Could you check a few things on this model? Use its own coordinates, in mm. A direction names the side the tool comes from. Coordinates: 2 decimals unless noted, no trailing zeros. Order: outer loops, then holes, each group sorted by start corner. A loop starts at its lowest first (then second) coordinate and runs counter-clockwise, first axis right, second up. Notation, with made-up numbers: (59.25, 54.25) - (82.25, 54.25) arc R17 cw to (82.25, 60.25) - close; hole circle Ø5 at (-37, -39.5). An arc over 180 degrees is marked (long way). One line per item, written item: value.
from build123d import *

# Parameters (mm, degrees)
SKETCH1_R                     = 43.815
HOUSING_FITTING_EXTRUDE_DEPTH = 17.018
HOUSING_BODY_1_DEPTH          = 25.4
SKETCH3_R                     = 6.3754
IMPELLER_BORE_DEPTH           = 17.018
O_RING_CUT_DEPTH              = 1.27
O_RING_CUT_DEPTH_BACK         = 1.27
SKETCH5_R                     = 43.942
SKETCH5_R_2                   = 43.18
SKETCH14_R                    = 3.3734375
CUT_EXTRUDE4_DEPTH            = 19.05
SKETCH15_R                    = 3.3734375
CUT_EXTRUDE5_DEPTH            = 19.05
FILLET1_R                     = 6.604
SKETCH20_R                    = 60.96
SKETCH20_R_2                  = 43.815
BOSS_EXTRUDE1_DEPTH           = 3.175
SKETCH21_R                    = 60.96
SKETCH21_R_2                  = 57.15
BOSS_EXTRUDE2_DEPTH           = 38.1
SKETCH23_R                    = 50.00625
SKETCH23_R_2                  = 43.815
BOSS_EXTRUDE3_DEPTH           = 13.843
SKETCH25_R                    = 3.3734375
CUT_EXTRUDE13_DEPTH           = 25.4
SKETCH26_R                    = 12.954
CUT_EXTRUDE14_DEPTH           = 25.908
SKETCH29_R                    = 45.72
SKETCH29_R_2                  = 44.45
SKETCH29_R_3                  = 43.18
SKETCH29_R_4                  = 41.91
SKETCH29_R_5                  = 40.64
SKETCH29_R_6                  = 39.37
SKETCH29_R_7                  = 38.1
SKETCH29_R_8                  = 36.83
SKETCH29_R_9                  = 35.56
SKETCH29_R_10                 = 34.29
SKETCH29_R_11                 = 33.02
SKETCH29_R_12                 = 31.75
SKETCH29_R_13                 = 30.48
SKETCH29_R_14                 = 29.21
SKETCH29_R_15                 = 27.94
SKETCH29_R_16                 = 26.67
SKETCH29_R_17                 = 25.4
CUT_EXTRUDE16_DEPTH           = 1.5875


with BuildPart() as part:
    # Sketch1 → Housing Fitting Extrude (new body)
    with BuildSketch(Plane(origin=(0, 0, 0), x_dir=(0, 0, -1), z_dir=(1, 0, 0))):
        Circle(SKETCH1_R)
    extrude(amount=HOUSING_FITTING_EXTRUDE_DEPTH)

    # Sketch2 → Housing Body 1 (add)
    with BuildSketch(Plane.ZY):
        with BuildLine():
            Line((60.96, 0), (60.96, 60.96))
            Line((60.96, 60.96), (0, 60.96))
            ThreePointArc((0, 60.96), (-43.105229381, 43.105229381), (-60.96, 0))
            Line((-60.96, 0), (-60.96, -54.61))
            Line((-60.96, -54.61), (-60.96, -60.96))
            Line((-60.96, -60.96), (60.96, -60.96))
            Line((60.96, -60.96), (60.96, -54.61))
            Line((60.96, -54.61), (60.96, 0))
        make_face()
    extrude(amount=HOUSING_BODY_1_DEPTH)

    # Sketch3 → Impeller Bore (cut)
    with BuildSketch(Plane(origin=(17.018, 0, 0), x_dir=(0, 0, -1), z_dir=(1, 0, 0))):
        Circle(SKETCH3_R)
    extrude(amount=-IMPELLER_BORE_DEPTH, mode=Mode.SUBTRACT)

    # Sketch5 → O-Ring Cut (cut, two sides: drawn at the far end of the back side and taken through both)
    with BuildSketch(Plane(origin=(8.509, 0, 0), x_dir=(0, 0, -1), z_dir=(1, 0, 0)).offset(-O_RING_CUT_DEPTH_BACK)):
        Circle(SKETCH5_R)
        Circle(SKETCH5_R_2, mode=Mode.SUBTRACT)
    extrude(amount=O_RING_CUT_DEPTH + O_RING_CUT_DEPTH_BACK, mode=Mode.SUBTRACT)

    # Sketch14 → Cut-Extrude4 (cut)
    with BuildSketch(Plane.XZ.offset(60.96)):
        with Locations(Location((-9.525, -41.91, 0), (0, 0, 270))):
            Circle(SKETCH14_R)
        with Locations(Location((-9.525, 41.91, 0), (0, 0, 270))):
            Circle(SKETCH14_R)
    extrude(amount=-CUT_EXTRUDE4_DEPTH, mode=Mode.SUBTRACT)

    # Sketch15 → Cut-Extrude5 (cut)
    with BuildSketch(Plane(origin=(0, 0, -60.96), x_dir=(-1, 0, 0), z_dir=(0, 0, -1))):
        with Locations(Location((9.525, -35.56, 0), (0, 0, 90))):
            Circle(SKETCH15_R)
    extrude(amount=-CUT_EXTRUDE5_DEPTH, mode=Mode.SUBTRACT)

    # Fillet1
    fillet1_edges = [part.edges().sort_by_distance(p)[0] for p in [
        (17.018, 0, 6.3754),
    ]]
    fillet(fillet1_edges, radius=FILLET1_R)

    # Sketch20 → Boss-Extrude1 (add)
    with BuildSketch(Plane(origin=(0, 0, 0), x_dir=(0, 0, -1), z_dir=(1, 0, 0))):
        Circle(SKETCH20_R)
        Circle(SKETCH20_R_2, mode=Mode.SUBTRACT)
    extrude(amount=BOSS_EXTRUDE1_DEPTH)

    # Sketch21 → Boss-Extrude2 (add)
    with BuildSketch(Plane(origin=(3.175, 0, 0), x_dir=(0, 0, -1), z_dir=(1, 0, 0))):
        Circle(SKETCH21_R)
        with Locations(Location((0, 0, 0), (0, 0, 180))):
            Circle(SKETCH21_R_2, mode=Mode.SUBTRACT)
    extrude(amount=BOSS_EXTRUDE2_DEPTH)

    # Sketch23 → Boss-Extrude3 (add)
    with BuildSketch(Plane(origin=(3.175, 0, 0), x_dir=(0, 0, -1), z_dir=(1, 0, 0))):
        Circle(SKETCH23_R)
        Circle(SKETCH23_R_2, mode=Mode.SUBTRACT)
    extrude(amount=BOSS_EXTRUDE3_DEPTH)

    # Sketch25 → Cut-Extrude13 (cut)
    with BuildSketch(Plane.ZY.offset(25.4)):
        with Locations((37.777249767, 4.948676591)):
            Circle(SKETCH25_R)
        with Locations((30.211792261, -23.21330671)):
            Circle(SKETCH25_R)
        with Locations((4.948676591, -37.777249767)):
            Circle(SKETCH25_R)
        with Locations((-23.21330671, -30.211792261)):
            Circle(SKETCH25_R)
        with Locations((-37.777249767, -4.948676591)):
            Circle(SKETCH25_R)
        with Locations((-30.211792261, 23.21330671)):
            Circle(SKETCH25_R)
        with Locations((-4.948676591, 37.777249767)):
            Circle(SKETCH25_R)
        with Locations((23.21330671, 30.211792261)):
            Circle(SKETCH25_R)
    extrude(amount=-CUT_EXTRUDE13_DEPTH, mode=Mode.SUBTRACT)

    # Sketch26 → Cut-Extrude14 (cut)
    with BuildSketch(Plane.ZY.offset(25.4)):
        Circle(SKETCH26_R)
    extrude(amount=-CUT_EXTRUDE14_DEPTH, mode=Mode.SUBTRACT)

    # Sketch29 → Cut-Extrude16 (cut)
    # profile 1 of 9: a face of its own
    with BuildSketch(Plane(origin=(17.018, 0, 0), x_dir=(0, 0, -1), z_dir=(1, 0, 0))):
        Circle(SKETCH29_R)
        Circle(SKETCH29_R_2, mode=Mode.SUBTRACT)
    # profile 2 of 9: a face of its own
    with BuildSketch(Plane(origin=(17.018, 0, 0), x_dir=(0, 0, -1), z_dir=(1, 0, 0))):
        Circle(SKETCH29_R_3)
        Circle(SKETCH29_R_4, mode=Mode.SUBTRACT)
    # profile 3 of 9: a face of its own
    with BuildSketch(Plane(origin=(17.018, 0, 0), x_dir=(0, 0, -1), z_dir=(1, 0, 0))):
        Circle(SKETCH29_R_5)
        Circle(SKETCH29_R_6, mode=Mode.SUBTRACT)
    # profile 4 of 9: a face of its own
    with BuildSketch(Plane(origin=(17.018, 0, 0), x_dir=(0, 0, -1), z_dir=(1, 0, 0))):
        Circle(SKETCH29_R_7)
        Circle(SKETCH29_R_8, mode=Mode.SUBTRACT)
    # profile 5 of 9: a face of its own
    with BuildSketch(Plane(origin=(17.018, 0, 0), x_dir=(0, 0, -1), z_dir=(1, 0, 0))):
        Circle(SKETCH29_R_9)
        Circle(SKETCH29_R_10, mode=Mode.SUBTRACT)
    # profile 6 of 9: a face of its own
    with BuildSketch(Plane(origin=(17.018, 0, 0), x_dir=(0, 0, -1), z_dir=(1, 0, 0))):
        Circle(SKETCH29_R_11)
        Circle(SKETCH29_R_12, mode=Mode.SUBTRACT)
    # profile 7 of 9: a face of its own
    with BuildSketch(Plane(origin=(17.018, 0, 0), x_dir=(0, 0, -1), z_dir=(1, 0, 0))):
        Circle(SKETCH29_R_13)
        Circle(SKETCH29_R_14, mode=Mode.SUBTRACT)
    # profile 8 of 9: a face of its own
    with BuildSketch(Plane(origin=(17.018, 0, 0), x_dir=(0, 0, -1), z_dir=(1, 0, 0))):
        Circle(SKETCH29_R_15)
        Circle(SKETCH29_R_16, mode=Mode.SUBTRACT)
    # profile 9 of 9: a face of its own
    with BuildSketch(Plane(origin=(17.018, 0, 0), x_dir=(0, 0, -1), z_dir=(1, 0, 0))):
        Circle(SKETCH29_R_17)
    extrude(amount=-CUT_EXTRUDE16_DEPTH, mode=Mode.SUBTRACT)


solid = part.part
Item 1: For faces 1 (the face through (0, 38, -5)), 2 (the face through (16.235, -24.796, 5.506)), which set-ups out of +Z, -Z, +X, -X, +Y, -Y let a thin tool reach every point of the face, with its end or its side?
Conclusion:
face 1: -X
face 2: +X
Item 2: I want a section at A-A on x = -20.5. Give the number of separate pieces and of enclosed holes in the cut face, then the cut area to 3 significant figures.
Conclusion:
separate pieces: 1
enclosed holes: 9
area: 13,300 mm²
Item 3: I want a section at C-C on x = 33.5. Please give me the cut outline in (y, z).
Conclusion:
outline: circle Ø121.92 at (0, 0); hole circle Ø114.3 at (0, 0)
Item 4: I'm going to push flat-ended pins straight in: pin 1 Ø5 at (y, z) = (26, 32) entering from +X; pin 2 Ø16.5 at (y, z) = (0, 0) entering from +X; pin 3 Ø5 at (x, y) = (22, 34) entering from +Z. Where does each tip first touch, or does it pass through?
Conclusion:
pin 1: x = 17.02
pin 2: x = 15.02
pin 3: z = 52.19
Item 5: If I drill on probe 1 along Y at (x, z) = (14, 42); probe 2 along Z at (x, y) = (4.5, -17.5); probe 3 along Y at (x, z) = (6, 0), over which ranges is the centre line in solid material (lowest first)?
Conclusion:
probe 1: -44.18 to -38.76, -27.14 to 27.14, 38.76 to 44.18
probe 2: -58.39 to -54.4, -46.84 to 46.84, 54.4 to 58.39
probe 3: -60.96 to -57.15, -50.01 to -6.38, 6.38 to 50.01, 57.15 to 60.96
Item 6: I want a section at D-D on x = 12.5. Please give me the cut outline in (y, z), then the cut area to 3 significant figures.
Conclusion:
outline: circle Ø121.92 at (0, 0); circle Ø100.01 at (0, 0); hole circle Ø114.3 at (0, 0); hole circle Ø13.43 at (0, 0)
area: 9,130 mm²
Item 7: I want a section at B-B on y = -52. Please give me the cut outline in (x, z) (3 decimals).
Conclusion:
outline: (-25.4, -60.96) - (0, -60.96) - (0, -31.814) - (41.275, -31.814) - (41.275, -23.709) - (3.175, -23.709) - (3.175, 23.709) - (41.275, 23.709) - (41.275, 31.814) - (0, 31.814) - (0, 60.96) - (-25.4, 60.96) - close; hole circle Ø6.747 at (-9.525, -41.91); hole circle Ø6.747 at (-9.525, 41.91)
Item 8: Thinking about a two-plate mould opening in Z: for faces 3 (the face through (-9.38, -38.93, -51.57)), 4 (the face through (15.43, 31.2, 19.9)), which applies, pulls with the +Z half, pulls with the -Z half, needs draft (parallel to the pull), parting line crosses it, or undercut?
Conclusion:
face 3: needs draft
face 4: undercut
